For this review, use the dimensioned drawing (mm, ordinates from the lowest corner) and the shaded views. A direction names the side the tool comes from. Give positions to 0.01 mm unless a question says otherwise; leave off trailing zeros. Order: outer loops, then holes, each group sorted by start corner. A loop starts at its lowest first (then second) coordinate and runs counter-clockwise, first axis right, second up.
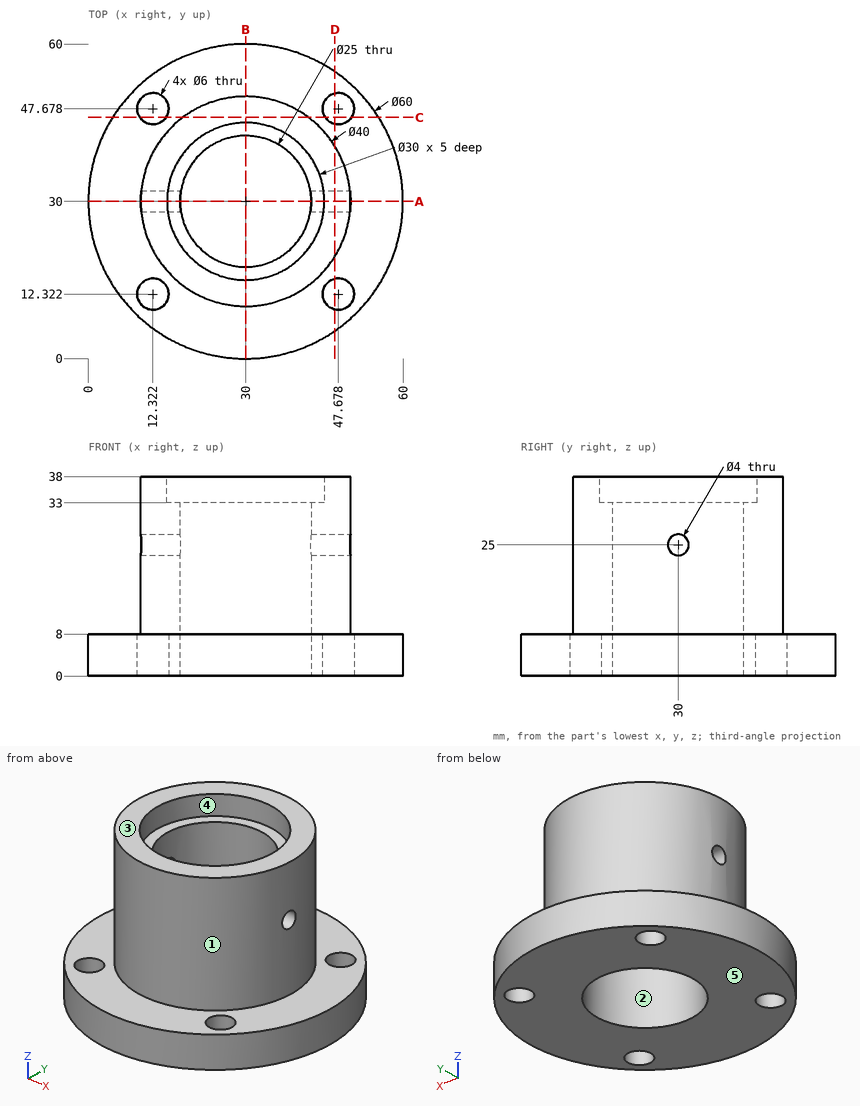
1. To check wall thickness, follow line 1 (Z direction, x = 50.5, y = 29); line 2 (X direction, y = 21.5, z = 10) (1 decimal); line 3 (Y direction, x = 33.5, z = 17.5). State the ranges of each line that lie inside material, in increasing order.
2. Draft analysis for pull direction Y (two halves, no side actions). For the marked faces 1, 2 and 3, state which applies: pulls with the +Y half, pulls with the -Y half, needs draft (parallel to the pull), parting line crosses it, or undercut.
3. Insertion check: pin 1 (4 mm diameter, centred on y = 29, z = 23, fed in from +X); pin 2 (1 mm diameter, centred on y = 42, z = 6, fed in from +X); pin 3 (18 mm diameter, centred on x = 34, y = 28.5, fed in from +Z). Each pin has a flat end and moves straight along its axis. Give the tip position at first contact, or say it passes through.
4. Take a section at C-C (y = 46). Write out the cut boundary in (x, z) (1 decimal), and give its area (3 significant figures).
5. Take a section at B-B (x = 30). Write out the cut boundary in (y, z), and give its area (3 significant figures).
6. For the marked faces 4 and 5, list the 3-axis set-ups (+Z, -Z, +X, -X, +Y, -Y) from which the entire face can be reached by the end or side of a thin tool; tool diameter is ignored.
7. Take a section at A-A (y = 30). Write out the cut boundary in (x, z).
8. Take a section at D-D (x = 47). Write out the cut boundary in (y, z) (1 decimal).
Answer:
1. line 1: z = 0 to 8
1. line 2: x = 11.9 to 20.8, 39.2 to 48.1
1. line 3: y = 10.31 to 18, 42 to 49.69
2. face 1: parting line crosses it
2. face 2: undercut
2. face 3: needs draft
3. pin 1: stops at x = 50
3. pin 2: stops at x = 57.71
3. pin 3: stops at z = 33
4. outline: (4.6, 0) - (9.8, 0) - (9.8, 8) - (4.6, 8) - close; (14.8, 0) - (45.2, 0) - (45.2, 8) - (42, 8) - (42, 38) - (18, 38) - (18, 8) - (14.8, 8) - close; (50.2, 0) - (55.4, 0) - (55.4, 8) - (50.2, 8) - close
4. area: 1,050 mm2
5. outline: (0, 0) - (17.5, 0) - (17.5, 33) - (15, 33) - (15, 38) - (10, 38) - (10, 8) - (0, 8) - close; (42.5, 0) - (60, 0) - (60, 8) - (50, 8) - (50, 38) - (45, 38) - (45, 33) - (42.5, 33) - close
5. area: 705 mm2
6. face 4: +Z
6. face 5: -Z, +X, -X, +Y, -Y
7. outline: (0, 0) - (17.5, 0) - (17.5, 23) - (10, 23) - (10, 8) - (0, 8) - close; (10, 27) - (17.5, 27) - (17.5, 33) - (15, 33) - (15, 38) - (10, 38) - close; (42.5, 0) - (60, 0) - (60, 8) - (50, 8) - (50, 23) - (42.5, 23) - close; (42.5, 27) - (50, 27) - (50, 38) - (45, 38) - (45, 33) - (42.5, 33) - close
8. outline: (5.3, 0) - (9.4, 0) - (9.4, 8) - (5.3, 8) - close; (15.2, 0) - (44.8, 0) - (44.8, 8) - (40.5, 8) - (40.5, 38) - (19.5, 38) - (19.5, 8) - (15.2, 8) - close; (50.6, 0) - (54.7, 0) - (54.7, 8) - (50.6, 8) - close; hole circle Ø4 at (30, 25)
